Source: CAD feature listing. Evaluate the final solid. Frame: model axes, mm. Face numbers are marked on the shaded views. A direction names the side the tool comes from. Give positions to 0.01 mm unless a question says otherwise; leave off trailing zeros. Order: outer loops, then holes, each group sorted by start corner. A loop starts at its lowest first (then second) coordinate and runs counter-clockwise, first axis right, second up. Notation, with made-up numbers: (82.5, 35) - (99.5, 35) arc R21 cw to (99.5, 48) - close; hole circle Ø1 at (88.5, 84.25). An arc over 180 degrees is marked (long way). Use CSV: the item, a comma, the result in double quotes.
```python
from build123d import *


with BuildPart() as part:
    # Sketch4 → Revolve5 (revolve)
    with BuildSketch(Plane.XY):
        with BuildLine():
            Line((50, 0), (30, 0))
            Line((30, 0), (30, -2.2))
            Line((30, -2.2), (49, -2.2))
            ThreePointArc((49, -2.2), (49.854727227, -1.261239649), (50, 0))
        make_face()
        Polygon((30, 0), (15, 0), (15, -2.925), (15, -3.15), (30, -3.15), (30, -2.2), align=None)
        with BuildLine():
            Line((15, 0), (-20, 0))
            ThreePointArc((-20, 0), (-21.025452167, -1.4625), (-20, -2.925))
            Line((-20, -2.925), (15, -2.925))
            Line((15, -2.925), (15, 0))
        make_face()
    revolve(axis=Axis((-50, 0, 0), (1, 0, 0)))


solid = part.part
```
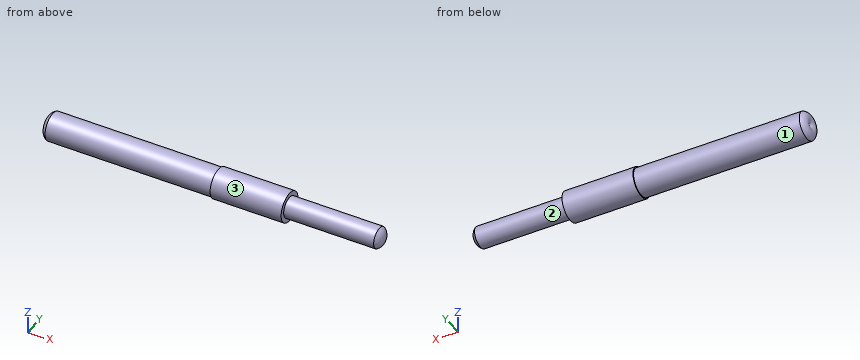
Item 1: Section B-B on x = 22.5. Return the cut outline in (y, z).
Filled in:
outline,"circle Ø6.3 at (0, 0)"
Item 2: Section A-A on x = 5. Return the cut outline in (y, z) (3 decimals).
Filled in:
outline,"circle Ø5.85 at (0, 0)"
Item 3: First-contact query: pin 1 (1.5 mm diameter, centred on x = -4, y = -2, fed in from +Z); pin 2 (1.5 mm diameter, centred on x = 20, z = -1.5, fed in from +Y); pin 3 (2 mm diameter, centred on x = 3, y = 2.5, fed in from +Z); pin 4 (1.9 mm diameter, centred on y = -0.5, z = 0.5, fed in from -X). Flat tips, straight axial feed; report the tip coordinate or a pass-through.
Filled in:
pin 1,"stops at z = 2.64"
pin 2,"stops at y = 3.06"
pin 3,"stops at z = 2.51"
pin 4,"stops at x = -21.03"
Item 4: Material intervals for line 1 (Y direction, x = 22, z = 0.25); line 2 (Y direction, x = -10, z = -0.25), sorted ascending. Write a range as from..to.
Filled in:
line 1,"y = -3.14..3.14"
line 2,"y = -2.91..2.91"
Item 5: Set-up query: the marked faces 1, 2 and 3. Return all of +Z, -Z, +X, -X, +Y, -Y with unobstructed straight access to the full face (end or side cutting, diameter ignored); none if empty.
Filled in:
face 1,"-X"
face 2,"+X"
face 3,"+X, -X"
